Verification items for the finished model (mm, model axes). A direction names the side the tool comes from. Round coordinates to 2 decimals unless told otherwise and drop trailing zeros. Write each loop counter-clockwise with the first axis right and the second up, starting at its lowest first coordinate (ties: lowest second). Pieces come first, ordered by that corner, then holes. Notation, with made-up numbers: (78.5, -22.5) - (114.5, -22.5) arc R23 ccw to (114.5, 1.5) - close; hole circle Ø4 at (71.5, 63). An arc over 180 degrees is marked (long way). Write each question's results on one line, items separated by ' | '.
```python
from build123d import *

# Parameters (mm, degrees)
CROQUIS1_R              = 1.5
CROQUIS1_R_2            = 0.5
SALIENTE_EXTRUIR1_DEPTH = 2.5


with BuildPart() as part:
    # Croquis1 → Saliente-Extruir1 (new body)
    with BuildSketch(Plane.XY):
        with BuildLine():
            Line((-25, -15), (-25, -5))
            ThreePointArc((-25, -5), (-19.142135624, 9.142135624), (-5, 15))
            Line((-5, 15), (5, 15))
            ThreePointArc((5, 15), (19.142135624, 9.142135624), (25, -5))
            Line((25, -5), (25, -15))
            Line((25, -15), (25, -27.5))
            Line((25, -27.5), (15, -27.5))
            Line((15, -27.5), (15, -30))
            Line((15, -30), (5, -30))
            Line((5, -30), (5, -27.5))
            Line((5, -27.5), (-5, -27.5))
            Line((-5, -27.5), (-5, -30))
            Line((-5, -30), (-15, -30))
            Line((-15, -30), (-15, -27.5))
            Line((-15, -27.5), (-25, -27.5))
            Line((-25, -27.5), (-25, -15))
        make_face()
        with Locations((-10, 10)):
            Circle(CROQUIS1_R, mode=Mode.SUBTRACT)
        with Locations((10, 10)):
            Circle(CROQUIS1_R, mode=Mode.SUBTRACT)
        with Locations((-10.5, -10)):
            Circle(CROQUIS1_R, mode=Mode.SUBTRACT)
        with Locations((10.5, -10)):
            Circle(CROQUIS1_R, mode=Mode.SUBTRACT)
        with Locations((15, -10)):
            Circle(CROQUIS1_R_2, mode=Mode.SUBTRACT)
        with Locations((6, -10)):
            Circle(CROQUIS1_R_2, mode=Mode.SUBTRACT)
    extrude(amount=SALIENTE_EXTRUIR1_DEPTH)


solid = part.part
```
(1) Go/stop test with flat-tipped pins: pin 1 Ø1.2 at (x, z) = (19, 2) entering from -Y; pin 2 Ø2.5 at (x, y) = (10, 10) entering from +Z; pin 3 Ø0.8 at (y, z) = (-28.5, 1) entering from +X; pin 4 Ø1.5 at (y, z) = (-3.5, 2) entering from -X. Record where each tip stops, or that it passes through.
Answer:
pin 1: y = -27.5 | pin 2: through | pin 3: x = 15 | pin 4: x = -24.99
(2) Set-up check for faces 4 (the flat face through (-15, -29, 1)), 5 (the flat face through (20, -27.5, 1)), 6 (the flat face through (0, -27.5, 1)), 7 (the cylindrical face through (-11.2, 9.1, 1.2)): record each of +Z, -Z, +X, -X, +Y, -Y from which the full face is reachable in a straight line by a thin tool's end or side.
Answer:
face 4: +Z, -Z, -X, -Y | face 5: +Z, -Z, +X, -Y | face 6: +Z, -Z, -Y | face 7: +Z, -Z
(3) Section check A-A (z = 1). Record the cut outline in (x, y), plus the area to 3 significant figures.
Answer:
outline: (-25, -27.5) - (-15, -27.5) - (-15, -30) - (-5, -30) - (-5, -27.5) - (5, -27.5) - (5, -30) - (15, -30) - (15, -27.5) - (25, -27.5) - (25, -5) arc R20 ccw to (5, 15) - (-5, 15) arc R20 ccw to (-25, -5) - close; hole circle Ø3 at (-10.5, -10); hole circle Ø3 at (-10, 10); hole circle Ø1 at (6, -10); hole circle Ø3 at (10, 10); hole circle Ø3 at (10.5, -10); hole circle Ø1 at (15, -10) | area: 1,970 mm2
(4) Thickness scan on L1, parallel to Y at x = -10.5, z = 0.95; L2, parallel to Y at x = -2, z = 1.45; L3, parallel to Y at x = 6, z = 1.55. Record the ranges inside material, lowest first.
Answer:
L1: -30 to -11.5, -8.5 to 8.59, 11.41 to 14.23 | L2: -27.5 to 15 | L3: -30 to -10.5, -9.5 to 14.97
(5) Section check D-D (x = -21). Record the cut outline in (y, z).
Answer:
outline: (-27.5, 0) - (7, 0) - (7, 2.5) - (-27.5, 2.5) - close
(6) Section check B-B (x = -10.5). Record the cut outline in (y, z), plus the area to 3 significant figures.
Answer:
outline: (-30, 0) - (-11.5, 0) - (-11.5, 2.5) - (-30, 2.5) - close; (-8.5, 0) - (8.59, 0) - (8.59, 2.5) - (-8.5, 2.5) - close; (11.41, 0) - (14.23, 0) - (14.23, 2.5) - (11.41, 2.5) - close | area: 96.0 mm2
(7) Section check C-C (x = 10). Record the cut outline in (y, z), plus the area to 3 significant figures.
Answer:
outline: (-30, 0) - (-11.41, 0) - (-11.41, 2.5) - (-30, 2.5) - close; (-8.59, 0) - (8.5, 0) - (8.5, 2.5) - (-8.59, 2.5) - close; (11.5, 0) - (14.36, 0) - (14.36, 2.5) - (11.5, 2.5) - close | area: 96.3 mm2
(8) Mould release check, pull along Y, two halves, no side actions. Record for faces 1 (the flat face through (0, -7, 2.5)), 2 (the cylindrical face through (-11.7, -10.9, 1.2)), 3 (the flat face through (0, 15, 1)): released by +Y, released by -Y, zero draft, split by the parting line, or undercut.
Answer:
face 1: zero draft | face 2: undercut | face 3: released by +Y
